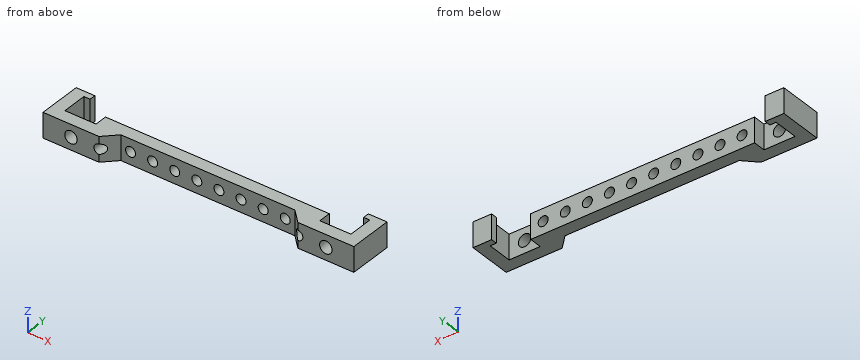
```python
from build123d import *

# Parameters (mm, degrees)
F0_W     = 16
F0_H     = 2
F0_W_2   = 2
F0_W_3   = 1
F0_H_2   = 1
F1_DEPTH = 4
F2_SIZE  = 1.99999
F3_R     = 1
F4_DEPTH = 2
F5_R     = 0.8008995453
F6_DEPTH = 5


# Not quite as in the source:
# - a fillet or chamfer is up to 0.001 mm smaller than in the source, because OpenCascade refuses the exact size


with BuildPart() as f1:
    # F0 (on Top) → F1 (new body)
    with BuildSketch(Plane.XY):
        with Locations((33, -4)):
            Rectangle(F0_W, F0_H)
        with Locations((17, -4)):
            Rectangle(F0_W, F0_H)
        Polygon((48, -5), (43, -5), (43, -7), (50, -7), (50, -5), align=None)
        with Locations((42, -6)):
            Rectangle(F0_W_2, F0_H)
        Polygon((2, -5), (0, -5), (0, -7), (7, -7), (7, -5), align=None)
        Polygon((2, 0), (0, 0), (0, -5), (2, -5), (2, -1), align=None)
        with Locations((47.5, -0.5)):
            Rectangle(F0_W_3, F0_H_2)
        with Locations((8, -4)):
            Rectangle(F0_W_2, F0_H)
        with Locations((8, -6)):
            Rectangle(F0_W_2, F0_H)
        with Locations((2.5, -0.5)):
            Rectangle(F0_W_3, F0_H_2)
        with Locations((42, -4)):
            Rectangle(F0_W_2, F0_H)
        Polygon((48, -1), (48, -5), (50, -5), (50, 0), (48, 0), align=None)
    extrude(amount=F1_DEPTH)

    # F2 (size 2 in the source; OpenCascade refuses exactly that, so slightly less here)
    f2_edges = [f1.edges().sort_by_distance(p)[0] for p in [
        (41, -5, 2),
        (9, -5, 2),
    ]]
    chamfer(f2_edges, length=F2_SIZE)

    # F3 (on face) → F4 (cut)
    with BuildSketch(Plane(origin=(0, -5, 0), x_dir=(-1, 0, 0), z_dir=(0, 1, 0))):
        with Locations((-4.5, 2)):
            Circle(F3_R)
        with Locations((-45.5, 2)):
            Circle(F3_R)
    extrude(amount=-F4_DEPTH, mode=Mode.SUBTRACT)

    # F5 (on face) → F6 (cut)
    with BuildSketch(Plane(origin=(0, -3, 0), x_dir=(-1, 0, 0), z_dir=(0, 1, 0))):
        with Locations((-16.1111111111, 2)):
            Circle(F5_R)
        with Locations((-9, 2)):
            Circle(F5_R)
        with Locations((-12.5555555556, 2)):
            Circle(F5_R)
        with Locations((-19.6666666667, 2)):
            Circle(F5_R)
        with Locations((-23.2222222222, 2)):
            Circle(F5_R)
        with Locations((-26.7777777778, 2)):
            Circle(F5_R)
        with Locations((-30.3333333333, 2)):
            Circle(F5_R)
        with Locations((-33.8888888889, 2)):
            Circle(F5_R)
        with Locations((-37.4444444444, 2)):
            Circle(F5_R)
        with Locations((-41, 2)):
            Circle(F5_R)
    extrude(amount=-F6_DEPTH, mode=Mode.SUBTRACT)


solid = f1.part
```
Here's how the part is built. I have some questions about the finished solid (model axes, mm). Round coordinates to 2 decimals unless told otherwise and drop trailing zeros. Write each loop counter-clockwise with the first axis right and the second up, starting at its lowest first coordinate (ties: lowest second). Pieces come first, ordered by that corner, then holes.
Q1. Will these pins go through, and if not, where does the flat tip stop? P1, Ø1.5, axis at x = 35.5, z = 3.5, coming from the +Y side; P2, Ø1.2, axis at y = -4, z = 2, coming from the -X side; P3, Ø1.2, axis at x = 5.5, z = 3, coming from the +Y side; P4, Ø2, axis at x = 16.11, z = 2, coming from the -Y side.
Q2. Please list where these lines run through material, in increasing order: probe 1 along X at (y, z) = (-4, 3.4); probe 2 along X at (y, z) = (-2, 2.45); probe 3 along Z at (x, y) = (41, -5.6).
Q3. If we section it at A-A on y = -4.5: Give the number of separate pieces and of enclosed holes in the cut face, plus the area to 3 significant figures.
Q4. If we section it at B-B on x = 4.5: Write out the boundary of the cut face in (y, z), plus the area to 3 significant figures.
Q5. If we section it at C-C on y = -2: Write out the boundary of the cut face in (x, z).
Answer below:
1. P1: stops at y = -3
1. P2: stops at x = 0
1. P3: stops at y = -5
1. P4: stops at y = -5
2. probe 1: x = 0 to 2, 7 to 43, 48 to 50
2. probe 2: x = 0 to 2, 48 to 50
2. probe 3: z = 0 to 1.2, 2.8 to 4
3. separate pieces: 3
3. enclosed holes: 10
3. area: 140 mm2
4. outline: (-7, 0) - (-5, 0) - (-5, 1) - (-7, 1) - close; (-7, 3) - (-5, 3) - (-5, 4) - (-7, 4) - close
4. area: 4.00 mm2
5. outline: (0, 0) - (2, 0) - (2, 4) - (0, 4) - close; (48, 0) - (50, 0) - (50, 4) - (48, 4) - close
